Here's how the part is built. I have some questions about the finished solid (model axes, mm). Coordinates: 2 decimals unless noted, no trailing zeros. Write each loop counter-clockwise with the first axis right and the second up, starting at its lowest first coordinate (ties: lowest second). Pieces come first, ordered by that corner, then holes.
Item 1: If we section it at B-B (y = 2.5): Please give me the cut outline in (x, z).
Item 2: If I drill on line 1 (X direction, y = -11, z = 1.1); line 2 (X direction, y = 2.5, z = 0.35); line 3 (X direction, y = -1, z = 1.3), over which ranges is the centre line in solid material (lowest first)?
Item 3: If we section it at C-C (z = 0.95): Count the separate pieces of the cut face and the enclosed holes in it, then the cut area to 3 significant figures.
Item 4: If we section it at A-A (x = -12.5): Please give me the cut outline in (y, z), then the cut area to 3 significant figures.
from build123d import *

# Parameters (mm, degrees)
F1_DEPTH = 1.5


# Not quite as in the source:
# - a feature names something its author has since deleted; it is built from what else it names


with BuildPart() as f1:
    # F0 (on Top) → F1 (new body)
    with BuildSketch(Plane.XY):
        with BuildLine():
            Line((-16.6795244343, 6.6792241971), (-17.9256127972, 7.6760931368))
            ThreePointArc((-17.9256127972, 7.6760931368), (-19.4817711686, 0.8429662711), (-18.5216556944, -6.0990384764))
            ThreePointArc((-18.5216556944, -6.0990384764), (-18.1379825879, -7.1598594707), (-17.6936088333, -8.1967192494))
            ThreePointArc((-17.6936088333, -8.1967192494), (-15.9787045712, -8.2544735786), (-15.1374953738, -9.75))
            ThreePointArc((-15.1374953738, -9.75), (-15.3526962413, -10.5907684717), (-15.9453715143, -11.2247551096))
            ThreePointArc((-15.9453715143, -11.2247551096), (-15.2696114831, -12.1280239592), (-14.5427501065, -12.9907051133))
            ThreePointArc((-14.5427501065, -12.9907051133), (0, -19.5), (14.5427501065, -12.9907051133))
            ThreePointArc((14.5427501065, -12.9907051133), (13.4233937587, -7.75), (18.5216556944, -6.0990384764))
            ThreePointArc((18.5216556944, -6.0990384764), (16.8874953738, 9.75), (3.978905588, 19.0897435897))
            ThreePointArc((3.978905588, 19.0897435897), (0, 15.5), (-3.978905588, 19.0897435897))
            ThreePointArc((-3.978905588, 19.0897435897), (-10.2620358256, 16.5813335023), (-15.3099476357, 12.0770651813))
            Line((-15.3099476357, 12.0770651813), (-13.4680928187, 9.5194474719))
            ThreePointArc((-13.4680928187, 9.5194474719), (-13.7890746093, 6.6466910805), (-16.6795244343, 6.6792241971))
        make_face()
        with BuildLine():
            ThreePointArc((4.2189837175, 12.7847634468), (11.2638316679, 13.3931361584), (11.8722043795, 6.348288208))
            Line((11.8722043795, 6.348288208), (7.846187435, 1.5611991336))
            ThreePointArc((7.846187435, 1.5611991336), (6.128355545, -5.1423008775), (-0.1750048611, -7.9980856021))
            Line((-0.1750048611, -7.9980856021), (-4.1902567902, -12.7942075969))
            ThreePointArc((-4.1902567902, -12.7942075969), (-11.2337204833, -13.4184024423), (-11.8579153287, -6.3749387493))
            Line((-11.8579153287, -6.3749387493), (-7.8426609809, -1.5788187794))
            ThreePointArc((-7.8426609809, -1.5788187794), (-6.128355545, 5.1423008775), (0.1929691871, 7.9976723422))
            Line((0.1929691871, 7.9976723422), (4.2189837175, 12.7847634468))
        make_face(mode=Mode.SUBTRACT)
        with BuildLine():
            ThreePointArc((-17.6936088333, -8.1967192494), (-18.1379825879, -7.1598594707), (-18.5216556944, -6.0990384764))
            ThreePointArc((-18.5216556944, -6.0990384764), (-19.2041408378, -6.4891483024), (-19.7971496554, -7.0052027467))
            ThreePointArc((-19.7971496554, -7.0052027467), (-19.2630878929, -8.3626218874), (-18.6360824437, -9.6796916868))
            ThreePointArc((-18.6360824437, -9.6796916868), (-18.36446034, -8.8113443184), (-17.6936088333, -8.1967192494))
        make_face()
        with BuildLine():
            ThreePointArc((-18.6360824437, -9.6796916868), (-19.2630878929, -8.3626218874), (-19.7971496554, -7.0052027467))
            ThreePointArc((-19.7971496554, -7.0052027467), (-20.3515969889, -11.75), (-15.965258365, -13.6422331507))
            ThreePointArc((-15.965258365, -13.6422331507), (-16.8737869432, -12.5010125269), (-17.7009001234, -11.2994749799))
            ThreePointArc((-17.7009001234, -11.2994749799), (-18.4030398304, -10.625), (-18.6360824437, -9.6796916868))
        make_face()
        with BuildLine():
            ThreePointArc((-14.5427501065, -12.9907051133), (-15.2696114831, -12.1280239592), (-15.9453715143, -11.2247551096))
            ThreePointArc((-15.9453715143, -11.2247551096), (-16.8130781912, -11.498417022), (-17.7009001234, -11.2994749799))
            ThreePointArc((-17.7009001234, -11.2994749799), (-16.8737869432, -12.5010125269), (-15.965258365, -13.6422331507))
            ThreePointArc((-15.965258365, -13.6422331507), (-15.2218376977, -13.3866996722), (-14.5427501065, -12.9907051133))
        make_face()
        with BuildLine():
            ThreePointArc((17.7009001234, -11.2994749799), (16.8737869432, -12.5010125269), (15.965258365, -13.6422331507))
            ThreePointArc((15.965258365, -13.6422331507), (19.3685286228, -12.8875904796), (20.8874953738, -9.75))
            ThreePointArc((20.8874953738, -9.75), (20.6049284348, -8.2732835625), (19.7971496554, -7.0052027467))
            ThreePointArc((19.7971496554, -7.0052027467), (19.2630878929, -8.3626218874), (18.6360824437, -9.6796916868))
            ThreePointArc((18.6360824437, -9.6796916868), (18.6371421056, -9.7148387455), (18.6374953738, -9.75))
            ThreePointArc((18.6374953738, -9.75), (18.3851532639, -10.6552739056), (17.7009001234, -11.2994749799))
        make_face()
        with BuildLine():
            ThreePointArc((14.5427501065, -12.9907051133), (15.2218376977, -13.3866996722), (15.965258365, -13.6422331507))
            ThreePointArc((15.965258365, -13.6422331507), (16.8737869432, -12.5010125269), (17.7009001234, -11.2994749799))
            ThreePointArc((17.7009001234, -11.2994749799), (16.8130781912, -11.498417022), (15.9453715143, -11.2247551096))
            ThreePointArc((15.9453715143, -11.2247551096), (15.2696114831, -12.1280239592), (14.5427501065, -12.9907051133))
        make_face()
        with BuildLine():
            ThreePointArc((-4, 19.5), (-3.994722916, 19.2946008177), (-3.978905588, 19.0897435897))
            ThreePointArc((-3.978905588, 19.0897435897), (-2.8683711048, 19.2878834299), (-1.748237319, 19.421474359))
            ThreePointArc((-1.748237319, 19.421474359), (-1.7495592743, 19.4607272889), (-1.75, 19.5))
            Line((-1.75, 19.5), (-4, 19.5))
        make_face()
        with BuildLine():
            ThreePointArc((-1.748237319, 19.421474359), (-2.8683711048, 19.2878834299), (-3.978905588, 19.0897435897))
            ThreePointArc((-3.978905588, 19.0897435897), (0, 15.5), (3.978905588, 19.0897435897))
            ThreePointArc((3.978905588, 19.0897435897), (2.8683711048, 19.2878834299), (1.748237319, 19.421474359))
            ThreePointArc((1.748237319, 19.421474359), (0, 17.75), (-1.748237319, 19.421474359))
        make_face()
        with BuildLine():
            ThreePointArc((18.5216556944, -6.0990384764), (13.4233937587, -7.75), (14.5427501065, -12.9907051133))
            ThreePointArc((14.5427501065, -12.9907051133), (15.2696114831, -12.1280239592), (15.9453715143, -11.2247551096))
            ThreePointArc((15.9453715143, -11.2247551096), (15.3719509172, -8.875), (17.6936088333, -8.1967192493))
            ThreePointArc((17.6936088333, -8.1967192493), (18.1379825879, -7.1598594707), (18.5216556944, -6.0990384764))
        make_face()
        with BuildLine():
            ThreePointArc((-3.8318912904, 20.6474358974), (-3.9577496865, 20.0798425814), (-4, 19.5))
            Line((-4, 19.5), (-1.75, 19.5))
            ThreePointArc((-1.75, 19.5), (-1.5328191447, 20.3443728263), (-0.9351823203, 20.9791666667))
            ThreePointArc((-0.9351823203, 20.9791666667), (-2.3893009497, 20.8636344143), (-3.8318912904, 20.6474358974))
        make_face()
        with BuildLine():
            ThreePointArc((1.748237319, 19.421474359), (2.8683711048, 19.2878834299), (3.978905588, 19.0897435897))
            ThreePointArc((3.978905588, 19.0897435897), (3.994722916, 19.2946008177), (4, 19.5))
            Line((4, 19.5), (1.75, 19.5))
            ThreePointArc((1.75, 19.5), (1.7495592743, 19.4607272889), (1.748237319, 19.421474359))
        make_face()
        with BuildLine():
            ThreePointArc((3.8318912904, 20.6474358974), (0, 23.5), (-3.8318912904, 20.6474358974))
            ThreePointArc((-3.8318912904, 20.6474358974), (-2.3893009497, 20.8636344143), (-0.9351823203, 20.9791666667))
            ThreePointArc((-0.9351823203, 20.9791666667), (0, 21.25), (0.9351823203, 20.9791666667))
            ThreePointArc((0.9351823203, 20.9791666667), (2.3893009497, 20.8636344143), (3.8318912904, 20.6474358974))
        make_face()
        with BuildLine():
            ThreePointArc((19.7971496554, -7.0052027467), (19.2041408378, -6.4891483024), (18.5216556944, -6.0990384764))
            ThreePointArc((18.5216556944, -6.0990384764), (18.1379825879, -7.1598594707), (17.6936088333, -8.1967192493))
            ThreePointArc((17.6936088333, -8.1967192493), (18.36446034, -8.8113443184), (18.6360824437, -9.6796916868))
            ThreePointArc((18.6360824437, -9.6796916868), (19.2630878929, -8.3626218874), (19.7971496554, -7.0052027467))
        make_face()
        with BuildLine():
            Line((1.75, 19.5), (4, 19.5))
            ThreePointArc((4, 19.5), (3.9577496865, 20.0798425814), (3.8318912904, 20.6474358974))
            ThreePointArc((3.8318912904, 20.6474358974), (2.3893009497, 20.8636344143), (0.9351823203, 20.9791666667))
            ThreePointArc((0.9351823203, 20.9791666667), (1.5328191447, 20.3443728263), (1.75, 19.5))
        make_face()
    extrude(amount=F1_DEPTH)


solid = f1.part
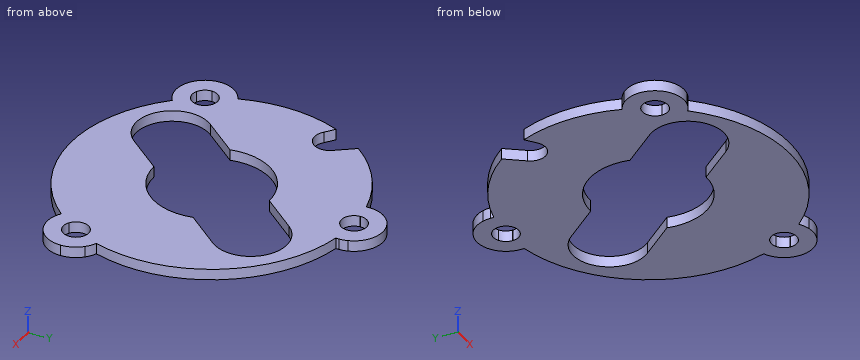
Answer list:
1. outline: (-19.34, 0) - (-7.6, 0) - (-7.6, 1.5) - (-19.34, 1.5) - close; (8.64, 0) - (19.34, 0) - (19.34, 1.5) - (8.64, 1.5) - close
2. line 1: x = -20.69 to -18.11, -15.66 to -12.82, -2.69 to 15.66, 18.11 to 20.69
2. line 2: x = -19.34 to -7.6, 8.64 to 19.34
2. line 3: x = -19.47 to -7.94, 7.94 to 19.47
3. separate pieces: 1
3. enclosed holes: 4
3. area: 846 mm2
4. outline: (-14.97, 0) - (-11.81, 0) - (-11.81, 1.5) - (-14.97, 1.5) - close; (-7.36, 0) - (14.97, 0) - (14.97, 1.5) - (-7.36, 1.5) - close
4. area: 38.2 mm2
